The listing builds one solid part. Answer for the finished solid, in the listing's coordinates (mm). A direction names the side the tool comes from. Give positions to 0.01 mm unless a question says otherwise; leave off trailing zeros. Order: outer loops, then holes, each group sorted by start corner. A loop starts at its lowest first (then second) coordinate and runs counter-clockwise, first axis right, second up.
```python
from build123d import *

# Parameters (mm, degrees)
SKETCH_1_W          = 40
SKETCH_1_H          = 60
SKETCH_1_R          = 1.5
EXTRUDE_1_DEPTH     = 3
FILLET_1_R          = 3
SKETCH_5_W          = 20
SKETCH_5_H          = 25
CUT_EXTRUDE_1_DEPTH = 38.89032563
FILLET_2_R          = 3


with BuildPart() as part:
    # 草图1 → 凸台-拉伸1 (new body)
    with BuildSketch(Plane(origin=(0, 0, 0), x_dir=(1, 0, 0), z_dir=(0, 1, 0))):
        with Locations((2.097965146, 0.632608651)):
            Rectangle(SKETCH_1_W, SKETCH_1_H)
        with Locations(Location((14.097965146, -25.367391349, 0), (0, 0, 270))):
            Circle(SKETCH_1_R, mode=Mode.SUBTRACT)
        with Locations(Location((-9.902034854, -25.367391349, 0), (0, 0, 270))):
            Circle(SKETCH_1_R, mode=Mode.SUBTRACT)
        with Locations(Location((14.097965146, -13.367391349, 0), (0, 0, 270))):
            Circle(SKETCH_1_R, mode=Mode.SUBTRACT)
        with Locations(Location((-9.902034854, -13.367391349, 0), (0, 0, 270))):
            Circle(SKETCH_1_R, mode=Mode.SUBTRACT)
        with Locations(Location((17.097965146, 2.632608651, 0), (0, 0, 270))):
            Circle(SKETCH_1_R, mode=Mode.SUBTRACT)
        with Locations(Location((-12.902034854, 2.632608651, 0), (0, 0, 270))):
            Circle(SKETCH_1_R, mode=Mode.SUBTRACT)
        with Locations(Location((17.097965146, 20.632608651, 0), (0, 0, 270))):
            Circle(SKETCH_1_R, mode=Mode.SUBTRACT)
        with Locations(Location((-12.902034854, 20.632608651, 0), (0, 0, 270))):
            Circle(SKETCH_1_R, mode=Mode.SUBTRACT)
    extrude(amount=EXTRUDE_1_DEPTH)

    # 圆角1
    fillet_1_edges = [part.edges().sort_by_distance(p)[0] for p in [
        (-17.902034854, 1.5, -30.632608651),
        (22.097965146, 1.5, -30.632608651),
        (22.097965146, 1.5, 29.367391349),
        (-17.902034854, 1.5, 29.367391349),
    ]]
    fillet(fillet_1_edges, radius=FILLET_1_R)

    # 草图5 → 切除-拉伸1 (cut, through all)
    with BuildSketch(Plane(origin=(0, 3, 0), x_dir=(1, 0, 0), z_dir=(0, 1, 0))):
        with Locations((2.097965146, 8.132608651)):
            Rectangle(SKETCH_5_W, SKETCH_5_H)
    extrude(amount=-CUT_EXTRUDE_1_DEPTH, mode=Mode.SUBTRACT)

    # 圆角2
    fillet_2_edges = [part.edges().sort_by_distance(p)[0] for p in [
        (-7.902034854, 1.5, 4.367391349),
        (-7.902034854, 1.5, -20.632608651),
        (12.097965146, 1.5, -20.632608651),
        (12.097965146, 1.5, 4.367391349),
    ]]
    fillet(fillet_2_edges, radius=FILLET_2_R)


solid = part.part
```
1) Straight lines are drawn through the part: probe 1 along Z at (x, y) = (17, 2.95); probe 2 along Z at (x, y) = (3.5, 0.5); probe 3 along X at (y, z) = (1.8, -16). For each, find the intervals that lie inside material, in ascending order.
Geometry says:
probe 1: z = -30.63 to -22.13, -19.14 to -4.13, -1.14 to 29.37
probe 2: z = -30.63 to -20.63, 4.37 to 29.37
probe 3: x = -17.9 to -7.9, 12.1 to 22.1
2) For a pull along Z with two mould halves and no side action, classify faces 3 (the cylindrical face through (12.767, 1.479, 14.06)), 4 (the cylindrical face through (21.196, 1.521, -29.777)), 5 (the flat face through (22.098, 1, 0)), 6 (the cylindrical face through (21.2, 1.52, 28.51)) as +Z half, -Z half, draft (parallel to the pull), parting line (faces both ways), or undercut.
Geometry says:
face 3: undercut
face 4: -Z half
face 5: draft
face 6: +Z half
3) Find section D-D (x = -10.5). Write down the section's boundary in (y, z), then the cut area to 3 significant figures.
Geometry says:
outline: (0, -30.63) - (3, -30.63) - (3, 11.99) - (0, 11.99) - close; (0, 14.74) - (3, 14.74) - (3, 23.99) - (0, 23.99) - close; (0, 26.74) - (3, 26.74) - (3, 29.37) - (0, 29.37) - close
area: 163 mm2
4) A tool of negligible diameter and unlimited length cuts with its end or side. For faces 1 (the flat face through (2, 2, -20.633)), 2 (the flat face through (2, 1, 29.367)), from which of +Z, -Z, +X, -X, +Y, -Y can it reach the whole face along a straight path? Write none if from no direction.
Geometry says:
face 1: +Y, -Y
face 2: +Z, +X, -X, +Y, -Y
5) Find section C-C (y = 1). Count the separate pieces of the cut face and the enclosed holes in it, then the cut area to 3 significant figures.
Geometry says:
separate pieces: 1
enclosed holes: 9
area: 1,840 mm2
6) Find section A-A (x = -3.5). Write down the section's boundary in (y, z), then the cut area to 3 significant figures.
Geometry says:
outline: (0, -30.63) - (3, -30.63) - (3, -20.63) - (0, -20.63) - close; (0, 4.37) - (3, 4.37) - (3, 29.37) - (0, 29.37) - close
area: 105 mm2
7) Find section B-B (z = -15). Write down the section's boundary in (x, y), then the cut area to 3 significant figures.
Geometry says:
outline: (-17.9, 0) - (-7.9, 0) - (-7.9, 3) - (-17.9, 3) - close; (12.1, 0) - (22.1, 0) - (22.1, 3) - (12.1, 3) - close
area: 60.0 mm2
8) Given P1, Ø2.5, axis at x = -9.9, z = 25.37, coming from the -Y side, flat-ended and moving along its own axis, determine where the tip first touches the part or whether it passes through.
Geometry says:
P1: passes through
